Design review of the part built by this model. Coordinates are the model's own, in mm. A direction names the side the tool comes from. Round coordinates to 2 decimals unless told otherwise and drop trailing zeros. Order: outer loops, then holes, each group sorted by start corner. A loop starts at its lowest first (then second) coordinate and runs counter-clockwise, first axis right, second up. Notation, with made-up numbers: (5.25, 82.5) - (29.25, 82.5) arc R33 cw to (29.25, 120.5) - close; hole circle Ø10 at (-23, 10). An arc over 180 degrees is marked (long way). Answer as a JSON object with one key per item and string values. Group by question number.
from build123d import *

# Parameters (mm, degrees)
QUADRADO_40_X_40_X_1_55_1_DEPTH = 578.0536
CORTE_EXTRUS_O1_DEPTH           = 293.466222183
CORTE_EXTRUS_O1_DEPTH_BACK      = 293.466222183
ESBO_O4_R                       = 3.5


with BuildPart() as part:
    # Esboço1 → Quadrado 40 X 40 X 1,55(1) (new body)
    with BuildSketch(Plane.YZ.offset(-289.0268)):
        with BuildLine():
            Line((-18, -20), (18, -20))
            ThreePointArc((18, -20), (19.414213562, -19.414213562), (20, -18))
            Line((20, -18), (20, 18))
            ThreePointArc((20, 18), (19.414213562, 19.414213562), (18, 20))
            Line((18, 20), (-18, 20))
            ThreePointArc((-18, 20), (-19.414213562, 19.414213562), (-20, 18))
            Line((-20, 18), (-20, -18))
            ThreePointArc((-20, -18), (-19.414213562, -19.414213562), (-18, -20))
        make_face()
        with BuildLine():
            Line((-18, -18.45), (18, -18.45))
            ThreePointArc((18, -18.45), (18.318198052, -18.318198052), (18.45, -18))
            Line((18.45, -18), (18.45, 18))
            ThreePointArc((18.45, 18), (18.318198052, 18.318198052), (18, 18.45))
            Line((18, 18.45), (-18, 18.45))
            ThreePointArc((-18, 18.45), (-18.318198052, 18.318198052), (-18.45, 18))
            Line((-18.45, 18), (-18.45, -18))
            ThreePointArc((-18.45, -18), (-18.318198052, -18.318198052), (-18, -18.45))
        make_face(mode=Mode.SUBTRACT)
    extrude(amount=QUADRADO_40_X_40_X_1_55_1_DEPTH)

    # Esboço4 → Corte-extrusão1 (cut, two sides: drawn at the far end of the back side and taken through both)
    with BuildSketch(Plane(origin=(0, 0, -20), x_dir=(-1, 0, 0), z_dir=(0, 0, -1)).offset(-CORTE_EXTRUS_O1_DEPTH_BACK)):
        with Locations(Location((-237.5, 0, 0), (0, 0, 270))):
            Circle(ESBO_O4_R)
        with Locations(Location((237.5, 0, 0), (0, 0, 270))):
            Circle(ESBO_O4_R)
    extrude(amount=CORTE_EXTRUS_O1_DEPTH + CORTE_EXTRUS_O1_DEPTH_BACK, mode=Mode.SUBTRACT)


solid = part.part
1. Take a section at C-C, the plane x = 181.5. Give the boundary of the cut face in (y, z).
2. Tool access review of faces 1 (the flat face through (-4, 0, -20)), 2 (the flat face through (-4, 0, -18.45)): name each direction out of +Z, -Z, +X, -X, +Y, -Y from which nothing blocks a thin tool from reaching the whole face with its end or side.
3. Take a section at A-A, the plane z = 8. Give the boundary of the cut face in (x, y), then the cut area to 3 significant figures.
4. Mouldability with a two-part tool opening along Y and no side actions: class faces 3 (the flat face through (-4, 20, 0)), 4 (the flat face through (-4, 0, 18.45)), 5 (the flat face through (-289.027, -2, -19)) as pulls with the +Y half, pulls with the -Y half, needs draft (parallel to the pull), parting line crosses it, or undercut.
5. To check wall thickness, follow line 1 (X direction, y = 0, z = 19.2); line 2 (Z direction, x = 26, y = -12). State the ranges of each line that lie inside material, in increasing order. Write a range as from..to.
Response values:
{
 "1": {"outline": "(-20, -18) arc R2 ccw to (-18, -20) - (18, -20) arc R2 ccw to (20, -18) - (20, 18) arc R2 ccw to (18, 20) - (-18, 20) arc R2 ccw to (-20, 18) - close; hole (-18.45, -18) arc R0.45 ccw to (-18, -18.45) - (18, -18.45) arc R0.45 ccw to (18.45, -18) - (18.45, 18) arc R0.45 ccw to (18, 18.45) - (-18, 18.45) arc R0.45 ccw to (-18.45, 18) - close"},
 "2": {"face 1": "-Z, +X, -X, +Y, -Y", "face 2": "+X, -X"},
 "3": {"outline": "(-289.03, -20) - (289.03, -20) - (289.03, -18.45) - (-289.03, -18.45) - close; (-289.03, 18.45) - (289.03, 18.45) - (289.03, 20) - (-289.03, 20) - close", "area": "1,790 mm2"},
 "4": {"face 3": "pulls with the +Y half", "face 4": "undercut", "face 5": "needs draft"},
 "5": {"line 1": "-289.03..-241, -234..234, 241..289.03", "line 2": "-20..-18.45, 18.45..20"}
}
